from build123d import *

# Parameters (mm, degrees)
BOSS_EXTRUDE1_DEPTH             = 0.762
SKETCH2_W                       = 22.352
SKETCH2_H                       = 13.5382
BOSS_EXTRUDE2_DEPTH             = 11.1125
SKETCH6_W                       = 12.0269
SKETCH6_H                       = 5.9055
CUT_EXTRUDE2_DEPTH              = 1.397
SKETCH3_W                       = 7.0866
SKETCH3_H                       = 5.5499
BOSS_EXTRUDE3_DEPTH             = 8.6106
BOSS_EXTRUDE3_DIRECTION_2_REACH = 41.105
FILLET4_SIZE                    = 3.5052
FILLET4_SIZE_2                  = 0.8382
SKETCH4_R                       = 1.318988248
CUT_EXTRUDE1_DEPTH              = 40.104844676
SKETCH5_W                       = 2.8194
SKETCH5_H                       = 0.6731
BOSS_EXTRUDE4_DEPTH             = 4.1021
FILLET5_RADIUS                  = 1.4097
FILLET5_LENGTH                  = 0.6731
FILLET6_RADIUS                  = 1.4097
FILLET6_LENGTH                  = 0.6731
FILLET7_RADIUS                  = 1.4097
FILLET7_LENGTH                  = 0.6731


with BuildPart() as part:
    # Sketch1 → Boss-Extrude1 (new body)
    with BuildSketch(Plane(origin=(0, 0, 0), x_dir=(1, 0, 0), z_dir=(0, 1, 0))):
        with BuildLine():
            Line((2.54, 0), (32.4231, 0))
            ThreePointArc((32.4231, 0), (34.219151224, 0.743948776), (34.9631, 2.54))
            Line((34.9631, 2.54), (34.9631, 10.9982))
            ThreePointArc((34.9631, 10.9982), (34.219151224, 12.794251224), (32.4231, 13.5382))
            Line((32.4231, 13.5382), (2.54, 13.5382))
            ThreePointArc((2.54, 13.5382), (0.743948776, 12.794251224), (0, 10.9982))
            Line((0, 10.9982), (0, 2.54))
            ThreePointArc((0, 2.54), (0.743948776, 0.743948776), (2.54, 0))
        make_face()
    extrude(amount=-BOSS_EXTRUDE1_DEPTH)

    # Sketch2 → Boss-Extrude2 (add)
    with BuildSketch(Plane(origin=(0, 0, 0), x_dir=(1, 0, 0), z_dir=(0, 1, 0))):
        with Locations((17.48155, 6.7691)):
            Rectangle(SKETCH2_W, SKETCH2_H)
    extrude(amount=-BOSS_EXTRUDE2_DEPTH)

    # Sketch6 → Cut-Extrude2 (cut)
    with BuildSketch(Plane(origin=(0, 0, 0), x_dir=(1, 0, 0), z_dir=(0, 1, 0))):
        with Locations((17.48155, 6.7691)):
            Rectangle(SKETCH6_W, SKETCH6_H)
    extrude(amount=-CUT_EXTRUDE2_DEPTH, mode=Mode.SUBTRACT)

    # Sketch3 → Boss-Extrude3 (add)
    with BuildSketch(Plane(origin=(0, 0, 0), x_dir=(1, 0, 0), z_dir=(0, 1, 0))):
        with Locations((15.0114, 6.7691)):
            Rectangle(SKETCH3_W, SKETCH3_H)
    extrude(amount=BOSS_EXTRUDE3_DEPTH)

    # Sketch3 → Boss-Extrude3 direction 2 (add, up to next)
    with BuildSketch(Plane(origin=(0, 0, 0), x_dir=(1, 0, 0), z_dir=(0, 1, 0)), mode=Mode.PRIVATE) as boss_extrude3_direction_2_sk1:
        with Locations((15.0114, 6.7691)):
            Rectangle(SKETCH3_W, SKETCH3_H)
    boss_extrude3_direction_2_tool1 = extrude(boss_extrude3_direction_2_sk1.sketch, amount=-BOSS_EXTRUDE3_DIRECTION_2_REACH, mode=Mode.PRIVATE) - part.part
    add(boss_extrude3_direction_2_tool1.solids().sort_by_distance((15.0114, 0, -6.7691))[0])

    # Fillet4
    # an asymmetric fillet: 3.5052, 0.8382 mm, written as the material it takes off along each edge
    with BuildSketch(Plane(origin=(18.5547, 8.6106, -18.30705), x_dir=(-1, 0, 0), z_dir=(0, 0, 1))) as fillet4_piece_1:
        with BuildLine():
            Bezier((FILLET4_SIZE, 0), (0, 0), (0, FILLET4_SIZE_2), weights=[1, 0.707106781, 1])
            Line((0, FILLET4_SIZE_2), (0, 0))
            Line((0, 0), (FILLET4_SIZE, 0))
        make_face()
    extrude(amount=23.0759, mode=Mode.SUBTRACT)
    with BuildSketch(Plane(origin=(11.4681, 8.6106, 4.76885), x_dir=(0, -1, 0), z_dir=(0, 0, -1))) as fillet4_piece_2:
        with BuildLine():
            Bezier((FILLET4_SIZE_2, 0), (0, 0), (0, -FILLET4_SIZE), weights=[1, 0.707106781, 1])
            Line((0, -FILLET4_SIZE), (0, 0))
            Line((0, 0), (FILLET4_SIZE_2, 0))
        make_face()
    extrude(amount=23.0759, mode=Mode.SUBTRACT)

    # Sketch4 → Cut-Extrude1 (cut, through all)
    with BuildSketch(Plane(origin=(0, 0, 0), x_dir=(1, 0, 0), z_dir=(0, 1, 0))):
        with Locations(Location((3.048, 6.7691, 0), (0, 0, 270))):
            Circle(SKETCH4_R)
        with Locations(Location((31.9151, 6.7691, 0), (0, 0, 270))):
            Circle(SKETCH4_R)
    extrude(amount=-CUT_EXTRUDE1_DEPTH, mode=Mode.SUBTRACT)

    # Sketch5 → Boss-Extrude4 (add)
    with BuildSketch(Plane.XZ.offset(11.1125)):
        with Locations((10.34415, -3.63855)):
            Rectangle(SKETCH5_W, SKETCH5_H)
        with Locations((17.48155, -3.63855)):
            Rectangle(SKETCH5_W, SKETCH5_H)
        with Locations((24.61895, -3.63855)):
            Rectangle(SKETCH5_W, SKETCH5_H)
    extrude(amount=BOSS_EXTRUDE4_DEPTH)

    # Fillet5: full round fillet: the end face becomes a half cylinder, R = half its width
    fillet5_face = Plane((10.34415, -15.2146, -3.63855), x_dir=(0, 0, -1), z_dir=(0, -1, 0))  # on the end face: x along it, z out of the body
    fillet5_slab = fillet5_face.offset(-FILLET5_RADIUS / 2) * Box(FILLET5_LENGTH, 2 * FILLET5_RADIUS, FILLET5_RADIUS, mode=Mode.PRIVATE)  # the body's end, R deep
    fillet5_round = Plane((10.34415, -13.8049, -3.63855), x_dir=(0, -1, 0), z_dir=(0, 0, -1)) * Cylinder(FILLET5_RADIUS, FILLET5_LENGTH, mode=Mode.PRIVATE)  # its axis R under the face
    add(fillet5_slab - fillet5_round, mode=Mode.SUBTRACT)

    # Fillet6: full round fillet: the end face becomes a half cylinder, R = half its width
    fillet6_face = Plane((17.48155, -15.2146, -3.63855), x_dir=(0, 0, -1), z_dir=(0, -1, 0))  # on the end face: x along it, z out of the body
    fillet6_slab = fillet6_face.offset(-FILLET6_RADIUS / 2) * Box(FILLET6_LENGTH, 2 * FILLET6_RADIUS, FILLET6_RADIUS, mode=Mode.PRIVATE)  # the body's end, R deep
    fillet6_round = Plane((17.48155, -13.8049, -3.63855), x_dir=(0, -1, 0), z_dir=(0, 0, -1)) * Cylinder(FILLET6_RADIUS, FILLET6_LENGTH, mode=Mode.PRIVATE)  # its axis R under the face
    add(fillet6_slab - fillet6_round, mode=Mode.SUBTRACT)

    # Fillet7: full round fillet: the end face becomes a half cylinder, R = half its width
    fillet7_face = Plane((24.61895, -15.2146, -3.63855), x_dir=(0, 0, -1), z_dir=(0, -1, 0))  # on the end face: x along it, z out of the body
    fillet7_slab = fillet7_face.offset(-FILLET7_RADIUS / 2) * Box(FILLET7_LENGTH, 2 * FILLET7_RADIUS, FILLET7_RADIUS, mode=Mode.PRIVATE)  # the body's end, R deep
    fillet7_round = Plane((24.61895, -13.8049, -3.63855), x_dir=(0, -1, 0), z_dir=(0, 0, -1)) * Cylinder(FILLET7_RADIUS, FILLET7_LENGTH, mode=Mode.PRIVATE)  # its axis R under the face
    add(fillet7_slab - fillet7_round, mode=Mode.SUBTRACT)


solid = part.part
Input: part model. Units: mm. Frame: model coordinates. A direction names the side the tool comes from. Give positions to 0.01 mm unless a question says otherwise; leave off trailing zeros. Order: outer loops, then holes, each group sorted by start corner. A loop starts at its lowest first (then second) coordinate and runs counter-clockwise, first axis right, second up. Notation, with made-up numbers: (43, 17) - (99, 17) arc R34 cw to (99, 55) - close; hole circle Ø8 at (7, 17.25). An arc over 180 degrees is marked (long way). Write each question's results on one line, items separated by ' | '.
Item 1: Section D-D (y = -9.25). Return loops of the section in (x, z).
A:
outline: (6.31, -13.54) - (28.66, -13.54) - (28.66, 0) - (6.31, 0) - close
Item 2: Section C-C (z = -12.25). Return loops of the section in (x, y).
A:
outline: (0.33, -0.76) - (6.31, -0.76) - (6.31, -11.11) - (28.66, -11.11) - (28.66, -0.76) - (34.63, -0.76) - (34.63, 0) - (0.33, 0) - close
Item 3: Material intervals for line 1 along X through (y, z) = (-12.25, -3.5); line 2 along X through (y, z) = (-8, -2.25); line 3 along Y through (x, z) = (22, -8), sorted ascending.
A:
line 1: x = 8.93 to 11.75, 16.07 to 18.89, 23.21 to 26.03 | line 2: x = 6.31 to 28.66 | line 3: y = -11.11 to -1.4
Item 4: Contact query for flat-ended pins moving along their axis: pin 1 Ø2.5 at (x, y) = (18, -14) entering from +Z; pin 2 Ø1.4 at (x, y) = (25, -14) entering from -Z; pin 3 Ø3 at (y, z) = (-4, -5) entering from -X; pin 4 Ø2 at (x, z) = (3.05, -6.77) entering from -Y. Output: stop coordinate, or through.
A:
pin 1: stops at z = -3.3 | pin 2: stops at z = -3.98 | pin 3: stops at x = 6.31 | pin 4: passes through
Item 5: Access query for faces 1 (the flat face through (25, -13, -3.302)), 2 (the flat face through (25, -13, -3.975)), 3 (the flat face through (11.468, 4, -7)), 4 (the flat face through (20, -1.397, -7)), 5 (the flat face through (5, -0.762, -7)). Directions: +Z, -Z, +X, -X, +Y, -Y. A direction counts if a zero-diameter tool reaches every point of the face in a straight line with its end or side. Return the directions, or none.
A:
face 1: +Z, +X, -X, -Y | face 2: -Z, +X, -X, -Y | face 3: +Z, -Z, -X, +Y | face 4: +Y | face 5: +Z, -Z, -X, -Y
Item 6: Section A-A (y = -13). Return loops of the section in (x, z), and give its area (3 significant figures).
A:
outline: (8.93, -3.98) - (11.75, -3.98) - (11.75, -3.3) - (8.93, -3.3) - close; (16.07, -3.98) - (18.89, -3.98) - (18.89, -3.3) - (16.07, -3.3) - close; (23.21, -3.98) - (26.03, -3.98) - (26.03, -3.3) - (23.21, -3.3) - close | area: 5.69 mm^2
Item 7: Section B-B (x = 4). Return loops of the section in (y, z).
A:
outline: (-0.76, -13.54) - (0, -13.54) - (0, -7.68) - (-0.76, -7.68) - close; (-0.76, -5.86) - (0, -5.86) - (0, 0) - (-0.76, 0) - close
